The drawing under review shows one solid part. Ordinate dimensions are in mm from its lowest x, y, z. A direction names the side the tool comes from. Give positions to 0.01 mm unless a question says otherwise; leave off trailing zeros. Order: outer loops, then holes, each group sorted by start corner. A loop starts at its lowest first (then second) coordinate and runs counter-clockwise, first axis right, second up. Notation, with made-up numbers: (75, -36.5) - (86, -36.5) arc R12 ccw to (86, -17.5) - close; hole circle Ø5 at (-1, -38). An arc over 180 degrees is marked (long way). Write item = value, one per line. Start each with the question number.
1. Wall thickness on probe 1 along X at (y, z) = (3, 6); probe 2 along Y at (x, z) = (3.5, 10); probe 3 along X at (y, z) = (12.1, 6): over which ranges is each line inside the solid? List them lowest first.
2. We need section D-D, the plane z = 3.5. Give the boundary of the cut face in (x, y).
3. We need section A-A, the plane x = 6. Give the boundary of the cut face in (y, z), and give its area (3 significant figures).
4. For P1, Ø5, axis at x = 6, z = 5, coming from the +Y side; P2, Ø6, axis at x = 8.5, y = 3, coming from the +Z side; P3, Ø6, axis at y = 6.5, z = 3.5, coming from the +X side, all flat-tipped, find the tip position at first contact; note any pin that passes through.
5. We need section B-B, the plane z = 6. Give the boundary of the cut face in (x, y), and give its area (3 significant figures).
6. We need section C-C, the plane y = 2.5. Give the boundary of the cut face in (x, z), and give its area (3 significant figures).
7. Mouldability with a two-part tool opening along Z and no side actions: class the marked faces 1, 2, 3 and 4 as pulls with the +Z half, pulls with the -Z half, needs draft (parallel to the pull), parting line crosses it, or undercut.
8. Machinability: for the marked faces 5 and 6, which of the approach directions +Z, -Z, +X, -X, +Y, -Y give a long, thin tool a straight path to every point of the face, cutting with its end or side? Answer none if there is none.
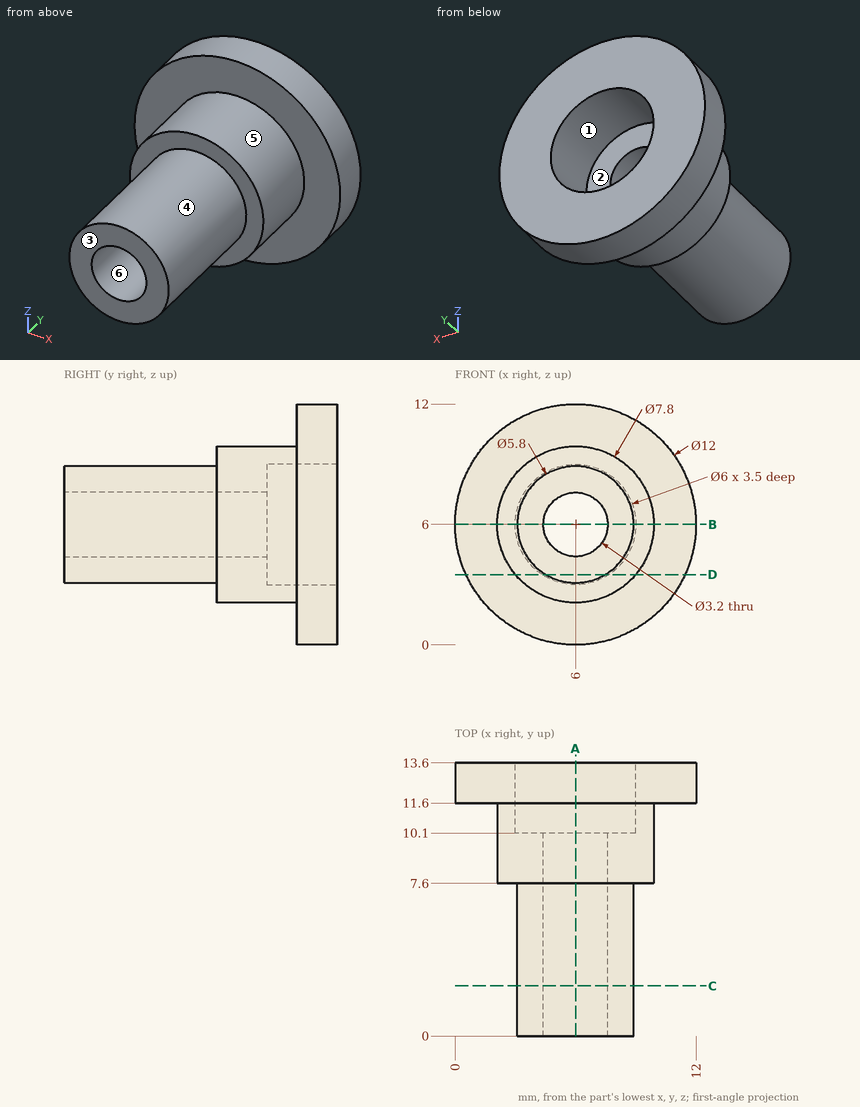
Model answer:
q1.probe_1 = 3.1 to 4.4, 7.6 to 8.9
q1.probe_2 = 11.6 to 13.6
q1.probe_3 = 0 to 3, 9 to 12
q2.outline = (0.55, 11.6) - (3.01, 11.6) - (3.01, 7.6) - (4.53, 7.6) - (4.53, 0) - (7.47, 0) - (7.47, 7.6) - (8.99, 7.6) - (8.99, 11.6) - (11.45, 11.6) - (11.45, 13.6) - (7.66, 13.6) - (7.66, 10.1) - (4.34, 10.1) - (4.34, 13.6) - (0.55, 13.6) - close
q3.outline = (0, 3.1) - (7.6, 3.1) - (7.6, 2.1) - (11.6, 2.1) - (11.6, 0) - (13.6, 0) - (13.6, 3) - (10.1, 3) - (10.1, 4.4) - (0, 4.4) - close; (0, 7.6) - (10.1, 7.6) - (10.1, 9) - (13.6, 9) - (13.6, 12) - (11.6, 12) - (11.6, 9.9) - (7.6, 9.9) - (7.6, 8.9) - (0, 8.9) - close
q3.area = 46.0 mm2
q4.P1 = 13.6
q4.P2 = 8.9
q4.P3 = 9.9
q5.outline = (0, 11.6) - (2.1, 11.6) - (2.1, 7.6) - (3.1, 7.6) - (3.1, 0) - (4.4, 0) - (4.4, 10.1) - (3, 10.1) - (3, 13.6) - (0, 13.6) - close; (7.6, 0) - (8.9, 0) - (8.9, 7.6) - (9.9, 7.6) - (9.9, 11.6) - (12, 11.6) - (12, 13.6) - (9, 13.6) - (9, 10.1) - (7.6, 10.1) - close
q5.area = 46.0 mm2
q6.outline = circle Ø5.8 at (6, 6); hole circle Ø3.2 at (6, 6)
q6.area = 18.4 mm2
q7.face_1 = undercut
q7.face_2 = undercut
q7.face_3 = needs draft
q7.face_4 = parting line crosses it
q8.face_5 = -Y
q8.face_6 = +Y, -Y
